```python
from build123d import *

# Parameters (mm, degrees)
SKETCH2_W             = 31.75
SKETCH2_H             = 31.75
BOSS_EXTRUDE1_DEPTH   = 508
BOSS_EXTRUDE1_2_DEPTH = 508
BOSS_EXTRUDE1_3_DEPTH = 508
BOSS_EXTRUDE1_4_DEPTH = 508
SKETCH3_W             = 1016
SKETCH3_H             = 1219.2
SKETCH3_W_2           = 952.5
SKETCH3_H_2           = 1155.7
BOSS_EXTRUDE2_DEPTH   = 31.75
BOSS_EXTRUDE3_START   = -457.2
SKETCH3_2_W           = 1016
SKETCH3_2_H           = 1219.2
SKETCH3_2_W_2         = 952.5
SKETCH3_2_H_2         = 1155.7
BOSS_EXTRUDE3_DEPTH   = 31.75
SKETCH4_W             = 100
SKETCH4_H             = 31.75
BOSS_EXTRUDE4_DEPTH   = 31.75
SKETCH5_W             = 31.75
SKETCH5_H             = 63.5
BOSS_EXTRUDE5_DEPTH   = 1155.7
SKETCH6_W             = 1016
SKETCH6_H             = 100
BOSS_EXTRUDE6_DEPTH   = 6.35


with BuildPart() as part:
    # Sketch2 → Boss-Extrude1 (new body)
    with BuildSketch(Plane(origin=(0, 0, 0), x_dir=(1, 0, 0), z_dir=(0, 1, 0))):
        with Locations((15.875, 1203.325)):
            Rectangle(SKETCH2_W, SKETCH2_H)
    extrude(amount=BOSS_EXTRUDE1_DEPTH)



with BuildPart() as body_2:
    # Sketch2 → Boss-Extrude1 2 (new body)
    with BuildSketch(Plane(origin=(0, 0, 0), x_dir=(1, 0, 0), z_dir=(0, 1, 0))):
        with Locations((15.875, 15.875)):
            Rectangle(SKETCH2_W, SKETCH2_H)
    extrude(amount=BOSS_EXTRUDE1_2_DEPTH)


with BuildPart() as body_3:
    # Sketch2 → Boss-Extrude1 3 (new body)
    with BuildSketch(Plane(origin=(0, 0, 0), x_dir=(1, 0, 0), z_dir=(0, 1, 0))):
        with Locations((1000.125, 15.875)):
            Rectangle(SKETCH2_W, SKETCH2_H)
    extrude(amount=BOSS_EXTRUDE1_3_DEPTH)


with BuildPart() as body_4:
    # Sketch2 → Boss-Extrude1 4 (new body)
    with BuildSketch(Plane(origin=(0, 0, 0), x_dir=(1, 0, 0), z_dir=(0, 1, 0))):
        with Locations((1000.125, 1203.325)):
            Rectangle(SKETCH2_W, SKETCH2_H)
    extrude(amount=BOSS_EXTRUDE1_4_DEPTH)


with BuildPart() as part_1:
    add(part.part)

    add(body_2.part)  # Boss-Extrude2 merges body 2

    add(body_3.part)  # Boss-Extrude2 merges body 3

    add(body_4.part)  # Boss-Extrude2 merges body 4
    # Sketch3 → Boss-Extrude2 (add)
    with BuildSketch(Plane(origin=(0, 508, 0), x_dir=(1, 0, 0), z_dir=(0, 1, 0))):
        with Locations((508, 609.6)):
            Rectangle(SKETCH3_W, SKETCH3_H)
        with Locations((508, 609.6)):
            Rectangle(SKETCH3_W_2, SKETCH3_H_2, mode=Mode.SUBTRACT)
    extrude(amount=BOSS_EXTRUDE2_DEPTH)

    # Sketch3<2> → Boss-Extrude3 (add)
    with BuildSketch(Plane(origin=(0, 508, 0), x_dir=(1, 0, 0), z_dir=(0, 1, 0)).offset(BOSS_EXTRUDE3_START)):
        with Locations((508, 609.6)):
            Rectangle(SKETCH3_2_W, SKETCH3_2_H)
        with Locations((508, 609.6)):
            Rectangle(SKETCH3_2_W_2, SKETCH3_2_H_2, mode=Mode.SUBTRACT)
    extrude(amount=BOSS_EXTRUDE3_DEPTH)

    # Sketch4 → Boss-Extrude4 (add)
    with BuildSketch(Plane(origin=(0, 539.75, 0), x_dir=(1, 0, 0), z_dir=(0, 1, 0))):
        with Locations((50, 1203.325)):
            Rectangle(SKETCH4_W, SKETCH4_H)
        with Locations((280, 1203.325)):
            Rectangle(SKETCH4_W, SKETCH4_H)
        with Locations((966, 1203.325)):
            Rectangle(SKETCH4_W, SKETCH4_H)
        with Locations((736, 1203.325)):
            Rectangle(SKETCH4_W, SKETCH4_H)
        with Locations((736, 15.875)):
            Rectangle(SKETCH4_W, SKETCH4_H)
        with Locations((966, 15.875)):
            Rectangle(SKETCH4_W, SKETCH4_H)
        with Locations((280, 15.875)):
            Rectangle(SKETCH4_W, SKETCH4_H)
        with Locations((50, 15.875)):
            Rectangle(SKETCH4_W, SKETCH4_H)
    extrude(amount=BOSS_EXTRUDE4_DEPTH)

    # Sketch5 → Boss-Extrude5 (add)
    with BuildSketch(Plane.XY.offset(-1187.45)):
        with Locations((84.125, 539.75)):
            Rectangle(SKETCH5_W, SKETCH5_H)
        with Locations((245.875, 539.75)):
            Rectangle(SKETCH5_W, SKETCH5_H)
        with Locations((770.125, 539.75)):
            Rectangle(SKETCH5_W, SKETCH5_H)
        with Locations((931.875, 539.75)):
            Rectangle(SKETCH5_W, SKETCH5_H)
    extrude(amount=BOSS_EXTRUDE5_DEPTH)

    # Sketch6 → Boss-Extrude6 (add)
    with BuildSketch(Plane(origin=(0, 0, -1219.2), x_dir=(-1, 0, 0), z_dir=(0, 0, -1))):
        with Locations((-508, 558)):
            Rectangle(SKETCH6_W, SKETCH6_H)
    extrude(amount=BOSS_EXTRUDE6_DEPTH)


solid = part_1.part
```
Check sheet for the modelled part. Datum: model origin and axes. Units: mm. A direction names the side the tool comes from. Give positions to 0.01 mm unless a question says otherwise; leave off trailing zeros. Order: outer loops, then holes, each group sorted by start corner. A loop starts at its lowest first (then second) coordinate and runs counter-clockwise, first axis right, second up. Notation, with made-up numbers: (24.5, 69.5) -> (83.5, 69.5) arc R32 cw to (83.5, 96.5) -> close; hole circle Ø10 at (-28, 73.25). An arc over 180 degrees is marked (long way). Return JSON: item names as keys, results as strings.
1. Cross-section at C-C, the plane y = 217.5. Record the cut outline in (x, z).
From the geometry:
{"outline": "(0, -1219.2) -> (31.75, -1219.2) -> (31.75, -1187.45) -> (0, -1187.45) -> close; (0, -31.75) -> (31.75, -31.75) -> (31.75, 0) -> (0, 0) -> close; (984.25, -1219.2) -> (1016, -1219.2) -> (1016, -1187.45) -> (984.25, -1187.45) -> close; (984.25, -31.75) -> (1016, -31.75) -> (1016, 0) -> (984.25, 0) -> close"}
2. Mould release check, pull along Z, two halves, no side actions. Record for faces 5 (the flat face through (1000, 508, -618)), 6 (the flat face through (984.25, 292, -1203)): +Z half, -Z half, draft (parallel to the pull), parting line (faces both ways), or undercut.
From the geometry:
{"face 5": "undercut", "face 6": "draft"}
3. Go/stop test with flat-tipped pins: P1, Ø16, axis at x = 1003, y = 14, coming from the -Z side; P2, Ø16, axis at x = 550.5, z = -14, coming from the +Y side. Record where each tip stops, or that it passes through.
From the geometry:
{"P1": "z = -1219.2", "P2": "y = 539.75"}
4. Cross-section at A-A, the plane x = 367.5. Record the cut outline in (y, z).
From the geometry:
{"outline": "(50.8, -1219.2) -> (82.55, -1219.2) -> (82.55, -1187.45) -> (50.8, -1187.45) -> close; (50.8, -31.75) -> (82.55, -31.75) -> (82.55, 0) -> (50.8, 0) -> close; (508, -1225.55) -> (608, -1225.55) -> (608, -1219.2) -> (539.75, -1219.2) -> (539.75, -1187.45) -> (508, -1187.45) -> close; (508, -31.75) -> (539.75, -31.75) -> (539.75, 0) -> (508, 0) -> close"}
5. Cross-section at B-B, the plane z = -76. Count the separate pieces of the cut face and the enclosed holes in it, plus the area to 3 significant figures.
From the geometry:
{"separate pieces": "8", "enclosed holes": "0", "area": "12,100 mm^2"}
6. Material ranges on probe 1 along X at (y, z) = (543.5, -684.5); probe 2 along X at (y, z) = (530, -115.5); probe 3 along Z at (x, y) = (351, 525.5), recorded low to high. Write a range as [from, to].
From the geometry:
{"probe 1": "[68.25, 100], [230, 261.75], [754.25, 786], [916, 947.75]", "probe 2": "[0, 31.75], [68.25, 100], [230, 261.75], [754.25, 786], [916, 947.75], [984.25, 1016]", "probe 3": "[-1225.55, -1187.45], [-31.75, 0]"}
7. Set-up check for faces 1 (the flat face through (68.25, 539, -618)), 2 (the flat face through (984.25, 25, -1203)), 3 (the flat face through (1000, 539.75, -618)), 4 (the flat face through (41, 546, -1187.45)): record each of +Z, -Z, +X, -X, +Y, -Y from which the full face is reachable in a straight line by a thin tool's end or side.
From the geometry:
{"face 1": "+Y, -Y", "face 2": "+Z, -Z, -Y", "face 3": "+X, +Y", "face 4": "+Y"}
